Could you check a few things on this drawing? It's one solid part, dimensions in mm from its lowest x, y, z. A direction names the side the tool comes from. Give positions to 0.01 mm unless a question says otherwise; leave off trailing zeros. Order: outer loops, then holes, each group sorted by start corner. A loop starts at its lowest first (then second) coordinate and runs counter-clockwise, first axis right, second up.
Item 1: I want a section at C-C, the plane z = 40. Write out the boundary of the cut face in (x, y), then the cut area to 3 significant figures.
Item 2: I want a section at B-B, the plane x = 30. Write out the boundary of the cut face in (y, z), then the cut area to 3 significant figures.
Item 3: Which directions (+Z, -Z, +X, -X, +Y, -Y) give clear straight access to the entire face, cutting with the end or side of a thin tool? Please do the marked faces 4 and 5.
Item 4: I want a section at A-A, the plane z = 56. Write out the boundary of the cut face in (x, y).
Item 5: If we mould it in two halves opening along Y, with no side actions, what happens to the marked faces 1, 2 and 3? For each: +Y half, -Y half, draft (parallel to the pull), parting line (faces both ways), or undercut.
Item 6: I want a section at D-D, the plane y = 15.5. Write out the boundary of the cut face in (x, z).
Item 7: I'm going to push flat-ended pins straight in: pin 1 Ø17.5 at (x, z) = (30, 40) entering from -Y; pin 2 Ø8 at (x, y) = (39, 54.5) entering from +Z. Where does each tip first touch, or does it pass through?
Item 8: If I drill on line 1 along Z through (x, y) = (30, 73.5); line 2 along X through (y, z) = (78, 40); line 3 along Y through (x, z) = (31, 51), over which ranges is the centre line in solid material (lowest first)?
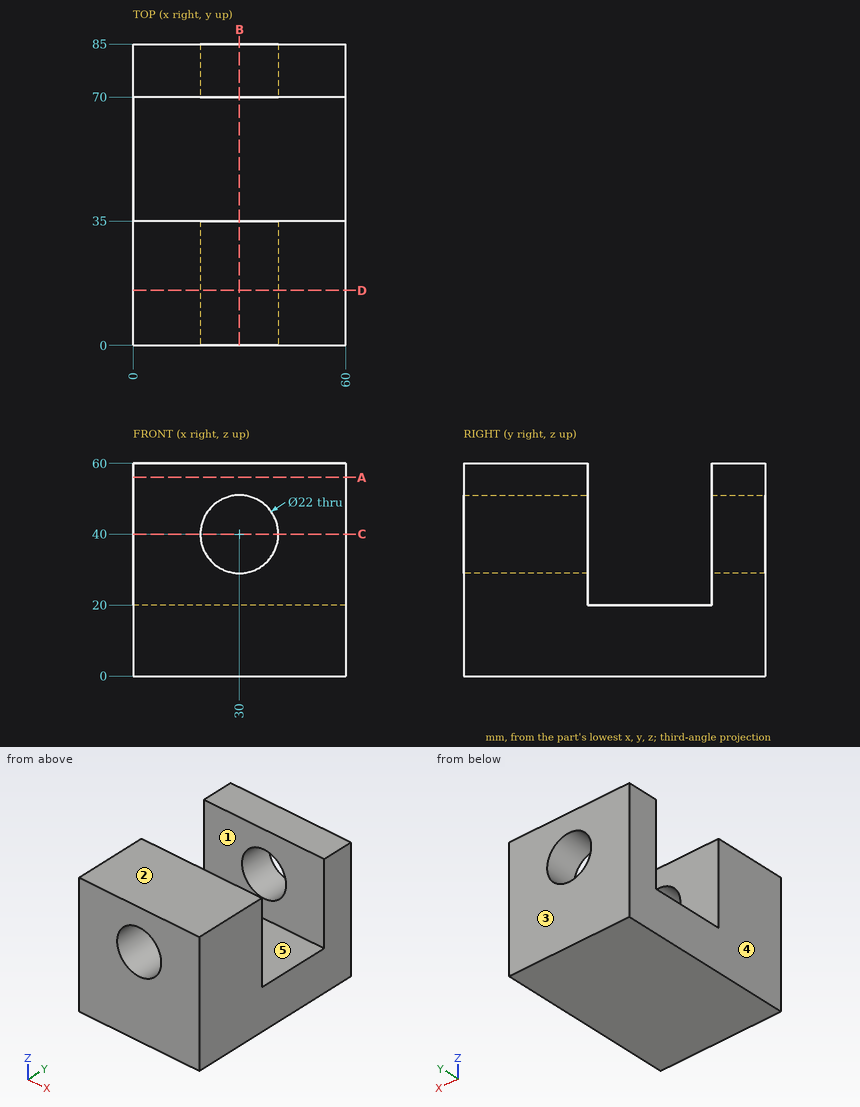
Results list:
1. outline: (0, 0) - (19, 0) - (19, 35) - (0, 35) - close; (0, 70) - (19, 70) - (19, 85) - (0, 85) - close; (41, 0) - (60, 0) - (60, 35) - (41, 35) - close; (41, 70) - (60, 70) - (60, 85) - (41, 85) - close
1. area: 1,900 mm2
2. outline: (0, 0) - (85, 0) - (85, 29) - (70, 29) - (70, 20) - (35, 20) - (35, 29) - (0, 29) - close; (0, 51) - (35, 51) - (35, 60) - (0, 60) - close; (70, 51) - (85, 51) - (85, 60) - (70, 60) - close
2. area: 2,600 mm2
3. face 4: +Z, -Z, -X, +Y, -Y
3. face 5: +Z, +X, -X
4. outline: (0, 0) - (60, 0) - (60, 35) - (0, 35) - close; (0, 70) - (60, 70) - (60, 85) - (0, 85) - close
5. face 1: undercut
5. face 2: draft
5. face 3: +Y half
6. outline: (0, 0) - (60, 0) - (60, 60) - (0, 60) - close; hole circle Ø22 at (30, 40)
7. pin 1: passes through
7. pin 2: stops at z = 20
8. line 1: z = 0 to 29, 51 to 60
8. line 2: x = 0 to 19, 41 to 60
8. line 3: y = 0 to 35, 70 to 85
